Here's the drawing with two shaded views (mm, measured from the low corner). I have some questions. Coordinates: 2 decimals unless noted, no trailing zeros. Write each loop counter-clockwise with the first axis right and the second up, starting at its lowest first coordinate (ties: lowest second). Pieces come first, ordered by that corner, then holes.
Item 1: If I drill on line 1 (Y direction, x = 2.2, z = 7.5) (3 decimals); line 2 (Y direction, x = 0.3, z = 34); line 3 (Z direction, x = 2.75, y = 31), over which ranges is the centre line in solid material (lowest first)?
Item 2: If we section it at C-C (z = 7.5): Please give me the cut outline in (x, y) (3 decimals), then the cut area to 3 significant figures.
Item 3: If we section it at D-D (x = 2.15): Please give me the cut outline in (y, z) (3 decimals).
Item 4: If we section it at A-A (z = 42): Please give me the cut outline in (x, y).
Item 5: I'm going to push a flat-ended pin straight in: pin 1 Ø4 at (y, z) = (13, 7.5) entering from -X. Where does the tip first touch, or does it pass through?
Item 6: If we section it at B-B (y = 13): Please give me the cut outline in (x, z) (3 decimals), then the cut area to 3 significant figures.
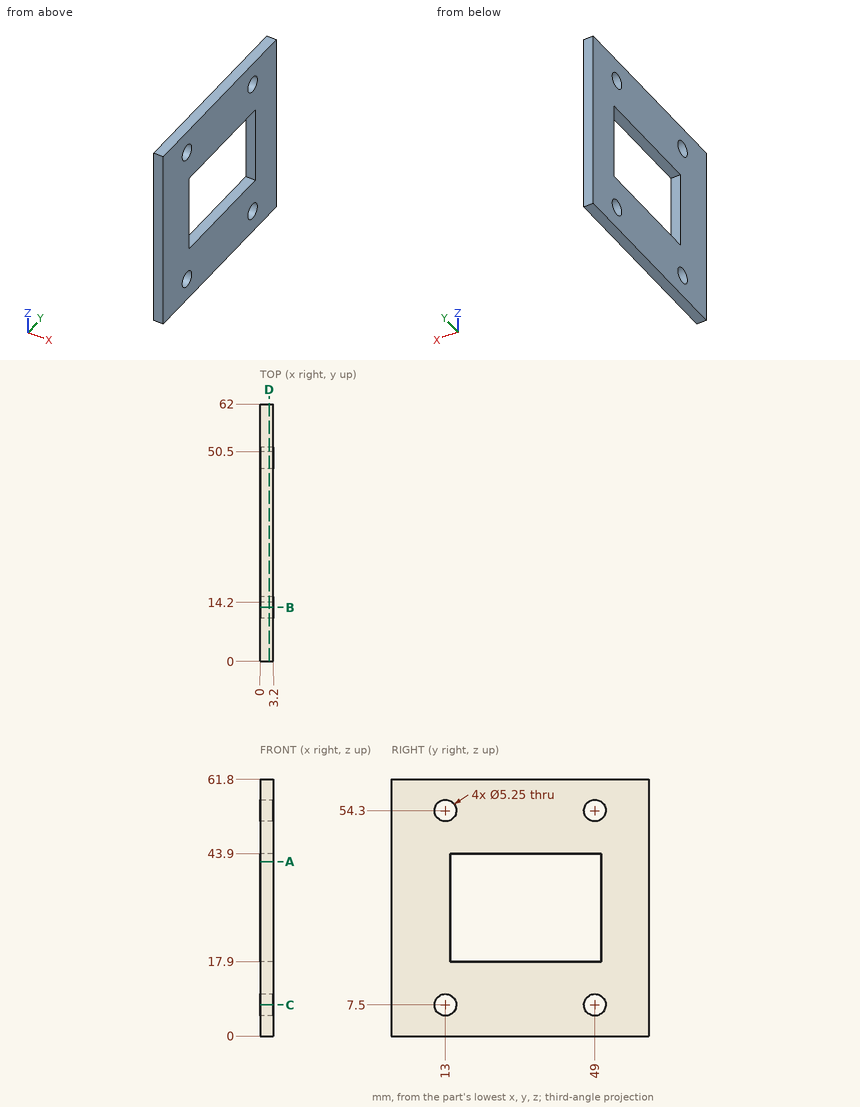
Answer list:
1. line 1: y = 0 to 10.375, 15.625 to 46.375, 51.625 to 62
1. line 2: y = 0 to 14.2, 50.5 to 62
1. line 3: z = 0 to 17.9, 43.9 to 61.8
2. outline: (0, 0) - (3.2, 0) - (3.2, 10.375) - (0, 10.375) - close; (0, 15.625) - (3.2, 15.625) - (3.2, 46.375) - (0, 46.375) - close; (0, 51.625) - (3.2, 51.625) - (3.2, 62) - (0, 62) - close
2. area: 165 mm2
3. outline: (0, 0) - (62, 0) - (62, 61.8) - (0, 61.8) - close; hole circle Ø5.25 at (13, 7.5); hole circle Ø5.25 at (13, 54.3); hole (14.2, 17.9) - (50.5, 17.9) - (50.5, 43.9) - (14.2, 43.9) - close; hole circle Ø5.25 at (49, 7.5); hole circle Ø5.25 at (49, 54.3)
4. outline: (0, 0) - (3.2, 0) - (3.2, 14.2) - (0, 14.2) - close; (0, 50.5) - (3.2, 50.5) - (3.2, 62) - (0, 62) - close
5. pin 1: passes through
6. outline: (0, 0) - (3.2, 0) - (3.2, 4.875) - (0, 4.875) - close; (0, 10.125) - (3.2, 10.125) - (3.2, 51.675) - (0, 51.675) - close; (0, 56.925) - (3.2, 56.925) - (3.2, 61.8) - (0, 61.8) - close
6. area: 164 mm2
